Autodesk Inventor part; units mm, degrees
ref_plane "YZ Plane" through (0, 0, 0) normal (1, 0, 0) x (0, 1, 0)
ref_plane "XZ Plane" through (0, 0, 0) normal (0, 1, 0) x (-1, 0, 0)
ref_plane "XY Plane" through (0, 0, 0) normal (0, 0, 1) x (1, 0, 0)
sketch "Sketch1" plane through (0, 0, 0) normal (0, 1, 0) x (-1, 0, 0)
  line L0 (0, 0) -> (28.575, 0)
  line L1 (28.575, 0) -> (0, 0)
  line L2 (0, 0) -> (-14.2875, -24.746676)
  line L3 (0, 0) -> (28.575, 0) construction
  line L4 (0, 0) -> (-14.2875, 24.746676)
  line L5 (0, 0) -> (28.575, 0) construction
  circle A0 centre (28.575, 0) radius 2.54
  circle A1 centre (-14.2875, -24.746676) radius 2.54
  circle A2 centre (-14.2875, 24.746676) radius 2.54
  circle A3 centre (0, 0) radius 3.175
  dimension "d0" = 28.575
  dimension "d1" = 28.575
  dimension "d2" = 120
  dimension "d3" = 28.575
  dimension "d4" = 120
  dimension "d5" = 5.08
  dimension "d6" = 5.08
  dimension "d7" = 5.08
  dimension "d9" = 6.35
sketch "Sketch2" plane through (0, 0, 0) normal (0, 1, 0) x (-1, 0, 0)
  circle A0 centre (28.575, 0) radius 2.54
  circle A1 centre (-14.2875, -24.746676) radius 2.54
  circle A2 centre (-14.2875, 24.746676) radius 2.54
  circle A3 centre (28.575, 0) radius 4.445
  circle A4 centre (-14.2875, -24.746676) radius 4.445
  circle A5 centre (-14.2875, 24.746676) radius 4.445
  circle A6 centre (0, 0) radius 6.35
  circle A7 centre (0, 0) radius 9.525
  line L0 (28.575, 4.445) -> (28.575, -4.445)
  line L1 (-14.2875, 24.746676) -> (0, 0)
  line L2 (0, 0) -> (-14.2875, 24.746676)
  line L3 (-14.2875, 24.746676) -> (-10.438017, 26.969176)
  line L4 (-14.2875, 24.746676) -> (-18.136983, 22.524176)
  line L5 (0, 0) -> (-14.2875, -24.746676)
  line L6 (-10.438017, -26.969176) -> (-14.2875, -24.746676)
  line L7 (-18.136983, -22.524176) -> (-14.2875, -24.746676)
  arc A8 (4.7625, 8.248892) -> (28.575, 4.445) centre (26.99693, 71.00172) ccw
  arc A9 (28.575, -4.445) -> (4.7625, -8.248892) centre (26.881025, -70.276152) ccw
  arc A10 (4.7625, -8.248892) -> (-10.438017, -26.969176) centre (47.42042, -58.417726) ccw
  arc A11 (-18.136983, -22.524176) -> (-9.525, 0) centre (-74.301445, 11.858426) ccw
  arc A12 (-9.525, 0) -> (-18.136983, 22.524176) centre (-78.365024, -13.41211) ccw
  arc A13 (-10.438017, 26.969176) -> (4.7625, 8.248892) centre (47.42042, 58.417726) ccw
  arc A14 (-3.701951, 16.907326) -> (16.495087, 5.259811) centre (24.822359, 43.03428) ccw
  arc A15 (16.493149, -5.24768) -> (-3.701951, -16.907326) centre (24.881633, -43.096252) ccw
  line L8 (-9.525, 0) -> (-10.9982, 0)
  arc A16 (-12.791199, -11.659646) -> (-12.855666, 11.634998) centre (-49.072802, -0.112643) ccw
  dimension "d10" = 8.89
  dimension "d11" = 8.89
  dimension "d12" = 8.89
  dimension "d13" = 12.7
  dimension "d14" = 19.05
  dimension "d15" = 1.4732
sketch "Sketch2 outline for Extrusion1" plane through (0, 0, 0) normal (0, 1, 0) x (-1, 0, 0)
  arc A0 (-10.438017, 26.969176) -> (-18.136983, 22.524176) centre (-14.2875, 24.746676) ccw
  arc A1 (-3.701951, 16.907326) -> (-10.438017, 26.969176) centre (47.42042, 58.417726) cw
  arc A2 (-18.136983, 22.524176) -> (-12.855666, 11.634998) centre (-78.365024, -13.41211) cw
  arc A3 (16.495087, 5.259811) -> (-3.701951, 16.907326) centre (24.822359, 43.03428) cw
  arc A4 (-12.855666, 11.634998) -> (-12.791199, -11.659646) centre (-49.072802, -0.112643) cw
  arc A5 (28.575, 4.445) -> (16.495087, 5.259811) centre (26.99693, 71.00172) cw
  arc A6 (-12.791199, -11.659646) -> (-18.136983, -22.524176) centre (-74.301445, 11.858426) cw
  arc A7 (28.575, -4.445) -> (28.575, 4.445) centre (28.575, 0) ccw
  arc A8 (-18.136983, -22.524176) -> (-10.438017, -26.969176) centre (-14.2875, -24.746676) ccw
  arc A9 (16.493149, -5.24768) -> (28.575, -4.445) centre (26.881025, -70.276152) cw
  arc A10 (-10.438017, -26.969176) -> (-3.701951, -16.907326) centre (47.42042, -58.417726) cw
  arc A11 (-3.701951, -16.907326) -> (16.493149, -5.24768) centre (24.881633, -43.096252) cw
  circle A12 centre (-14.2875, -24.746676) radius 2.54
  circle A13 centre (-14.2875, 24.746676) radius 2.54
  circle A14 centre (28.575, 0) radius 2.54
extrude "Extrusion1" add sketch "Sketch2 outline for Extrusion1" along normal blind 12.7
hole "Hole1" at (0, 0, 0) direction (0, 1, 0) diameter 6.35 end through all
sketch "Sketch3" plane through (0, 12.7, 0) normal (0, 1, 0) x (1, 0, 0)
  circle A0 centre (0, 0) radius 3.175
hole "Hole2" at (0, 12.7, 0) direction (0, -1, 0) diameter 6.604 end through all
properties part number "stability"
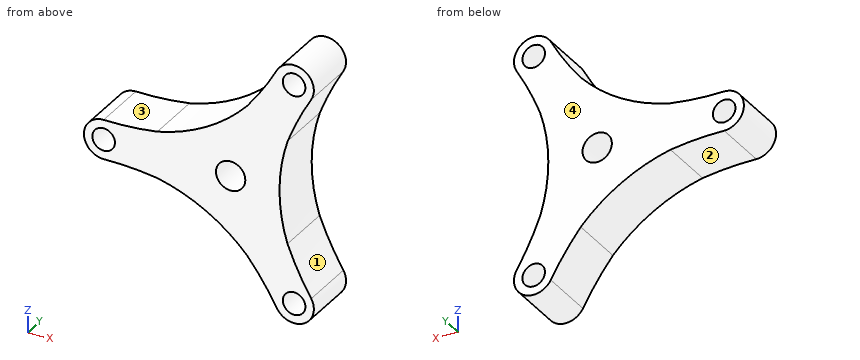
Model file for the job. Use its own axes, mm. Face numbers are marked on the shaded views. Give positions to 0.01 mm unless a question says otherwise; leave off trailing zeros. Loops run counter-clockwise (first coordinate to the right, second up) from the corner with the lowest first, then second, coordinate; pieces in that order, holes last. Notation, with made-up numbers: (46.25, 41) - (84.25, 41) arc R31 cw to (84.25, 74) - close; hole circle Ø1 at (5.5, 71). An arc over 180 degrees is marked (long way). One line per item, written item: value. Start each with the question number.
1. Slice it at D-D (y = 6.25). List the corners of the cut face in (x, z) (1 decimal), plus the area to 3 significant figures.
2. Slice it at A-A (z = 0). List the corners of the cut face in (x, y) (3 decimals), plus the area to 3 significant figures.
3. Slice it at C-C (x = 0). List the corners of the cut face in (y, z).
4. Pin check, flat tips, straight feed: pin 1 (1.5 mm diameter, centred on x = -24.5, y = 3, fed in from -Z); pin 2 (3 mm diameter, centred on y = 4.5, z = -2, fed in from +X); pin 3 (2 mm diameter, centred on y = 8, z = 21, fed in from +X); pin 4 (8 mm diameter, centred on x = -28.575, z = 0, fed in from -Y). Stop position of each tip, or through.
5. Pull direction Z, two halves, no side cores. Call the marked faces 1, 2, 3 and 4: pulls with the +Z half, pulls with the -Z half, needs draft (parallel to the pull), parting line crosses it, or undercut.
6. Probe L1, parallel to X at y = 3.75, z = -26; L2, parallel to Z at x = -26, y = 11; L3, parallel to X at y = 10, z = -23. List the from-to ranges inside material, lowest first. Write a range as from..to.
7. Slice it at B-B (x = 14). List the corners of the cut face in (y, z).
Solution:
1. outline: (-28.6, -4.4) arc R65.9 cw to (-16.5, -5.2) arc R38.8 cw to (3.7, -16.9) arc R65.9 cw to (10.4, -27) arc R4.4 ccw to (18.1, -22.5) arc R65.9 cw to (12.8, -11.7) arc R38.1 cw to (12.9, 11.6) arc R70.1 cw to (18.1, 22.5) arc R4.4 ccw to (10.4, 27) arc R65.9 cw to (3.7, 16.9) arc R38.7 cw to (-16.5, 5.3) arc R66.6 cw to (-28.6, 4.4) arc R4.4 ccw to start; hole circle Ø5.1 at (-28.6, 0); hole circle Ø6.6 at (0, 0); hole circle Ø5.1 at (14.3, -24.7); hole circle Ø5.1 at (14.3, 24.7)
1. area: 960 mm^2
2. outline: (-33.02, 0) - (-31.115, 0) - (-31.115, 12.7) - (-33.02, 12.7) - close; (-26.035, 0) - (-3.302, 0) - (-3.302, 12.7) - (-26.035, 12.7) - close; (3.302, 0) - (10.998, 0) - (10.998, 12.7) - (3.302, 12.7) - close
2. area: 411 mm^2
3. outline: (0, -13.37) - (12.7, -13.37) - (12.7, -3.3) - (0, -3.3) - close; (0, 3.3) - (12.7, 3.3) - (12.7, 13.37) - (0, 13.37) - close
4. pin 1: stops at z = -4.5
4. pin 2: stops at x = 11.15
4. pin 3: stops at x = 17.83
4. pin 4: stops at y = 0
5. face 1: undercut
5. face 2: pulls with the -Z half
5. face 3: pulls with the +Z half
5. face 4: needs draft
6. L1: x = 9.9..12.08, 16.5..18.55
6. L2: z = -4.43..4.43
6. L3: x = 8.1..12.44, 16.13..18.37
7. outline: (0, -29.18) - (12.7, -29.18) - (12.7, -27.27) - (0, -27.27) - close; (0, -22.22) - (12.7, -22.22) - (12.7, -14.61) - (0, -14.61) - close; (0, 14.44) - (12.7, 14.44) - (12.7, 22.22) - (0, 22.22) - close; (0, 27.27) - (12.7, 27.27) - (12.7, 29.18) - (0, 29.18) - close
